Geometry: final body of the model. Coordinates: model frame, mm. A direction names the side the tool comes from. Coordinates: 2 decimals unless noted, no trailing zeros. Write each loop counter-clockwise with the first axis right and the second up, starting at its lowest first coordinate (ties: lowest second). Pieces come first, ordered by that corner, then holes. Notation, with made-up numbers: (27.25, 78.25) - (62.25, 78.25) arc R13 cw to (62.25, 85.25) - close; hole circle Ø3 at (-15.75, 18). An arc over 180 degrees is marked (long way). Put each result on its own line as item: value.
```python
from build123d import *

# Parameters (mm, degrees)
ESQUISSE5_W         = 84
ESQUISSE5_H         = 56
BOSS_EXTRU_6_DEPTH  = 1.6
ESQUISSE6_W         = 77
ESQUISSE6_H         = 54
BOSS_EXTRU_8_DEPTH  = 3.5
ESQUISSE8_W         = 4
ESQUISSE8_H         = 6
BOSS_EXTRU_10_DEPTH = 1.5
ESQUISSE7_W         = 4
ESQUISSE7_H         = 6
BOSS_EXTRU_11_DEPTH = 1.5
ESQUISSE11_W        = 4
ESQUISSE11_H        = 6
BOSS_EXTRU_12_DEPTH = 1.5


with BuildPart() as part:
    # Esquisse5 → Boss.-Extru.6 (new body)
    with BuildSketch(Plane.XY):
        with Locations((42, 28)):
            Rectangle(ESQUISSE5_W, ESQUISSE5_H)
    extrude(amount=BOSS_EXTRU_6_DEPTH)

    # Esquisse6 → Boss.-Extru.8 (add)
    with BuildSketch(Plane(origin=(0, 0, 0), x_dir=(-1, 0, 0), z_dir=(0, 0, -1))):
        with Locations((-39.5, 28)):
            Rectangle(ESQUISSE6_W, ESQUISSE6_H)
    extrude(amount=BOSS_EXTRU_8_DEPTH)

    # Esquisse8 → Boss.-Extru.10 (add)
    with BuildSketch(Plane(origin=(0, 0, 0), x_dir=(-1, 0, 0), z_dir=(0, 0, -1))):
        with Locations((-81, 26)):
            Rectangle(ESQUISSE8_W, ESQUISSE8_H)
    extrude(amount=BOSS_EXTRU_10_DEPTH)

    # Esquisse7 → Boss.-Extru.11 (add)
    with BuildSketch(Plane(origin=(0, 0, 0), x_dir=(-1, 0, 0), z_dir=(0, 0, -1))):
        with Locations((-81, 39)):
            Rectangle(ESQUISSE7_W, ESQUISSE7_H)
    extrude(amount=BOSS_EXTRU_11_DEPTH)

    # Esquisse11 → Boss.-Extru.12 (add)
    with BuildSketch(Plane(origin=(0, 0, 0), x_dir=(-1, 0, 0), z_dir=(0, 0, -1))):
        with Locations((-81, 13)):
            Rectangle(ESQUISSE11_W, ESQUISSE11_H)
    extrude(amount=BOSS_EXTRU_12_DEPTH)


solid = part.part
```
1. Section query D-D (y = 14). Return loops of the section in (x, z).
Answer below:
outline: (0, 0) - (1, 0) - (1, -3.5) - (78, -3.5) - (78, 0) - (79, 0) - (79, -1.5) - (83, -1.5) - (83, 0) - (84, 0) - (84, 1.6) - (0, 1.6) - close
2. Section query A-A (y = 51.5). Return loops of the section in (x, z).
Answer below:
outline: (0, 0) - (1, 0) - (1, -3.5) - (78, -3.5) - (78, 0) - (84, 0) - (84, 1.6) - (0, 1.6) - close
3. Mould query, pull axis X, two halves, no side actions, for faces 4 (the flat face through (1, 28, -2)), 5 (the flat face through (78, 28, -2)), 6 (the flat face through (41, 28, 1.6)). Classes: +X half, -X half, draft (parallel to the pull), parting line (faces both ways), or undercut.
Answer below:
face 4: -X half
face 5: undercut
face 6: draft
4. Section query B-B (x = 51.5). Return loops of the section in (y, z), then the cut area to 3 significant figures.
Answer below:
outline: (0, 0) - (1, 0) - (1, -3.5) - (55, -3.5) - (55, 0) - (56, 0) - (56, 1.6) - (0, 1.6) - close
area: 279 mm²
5. Set-up query: faces 1 (the flat face through (40, 1, -2)), 2 (the flat face through (40, 55, -2)), 3 (the flat face through (81, 39, -1.5)). Return all of +Z, -Z, +X, -X, +Y, -Y with unobstructed straight access to the full face (end or side cutting, diameter ignored); none if empty.
Answer below:
face 1: -Z, +X, -X, -Y
face 2: -Z, +X, -X, +Y
face 3: -Z, +X, +Y, -Y
6. Section query C-C (z = -2.45). Return loops of the section in (x, y), then the cut area to 3 significant figures.
Answer below:
outline: (1, 1) - (78, 1) - (78, 55) - (1, 55) - close
area: 4,160 mm²
7. Ray query, probe 1 along X at (y, z) = (39.5, -0.6); probe 2 along Y at (x, z) = (63, -0.5); probe 3 along X at (y, z) = (35, -1). Return the intervals inside material, ascending. Write a range as from..to.
Answer below:
probe 1: x = 1..78, 79..83
probe 2: y = 1..55
probe 3: x = 1..78
8. Pin query (flat end, axial travel): pin 1 Ø1 at (x, z) = (45, -2) entering from -Y; pin 2 Ø1 at (y, z) = (19.5, -2) entering from +X; pin 3 Ø4.5 at (x, y) = (80.5, 26) entering from -Z. Return the tip coordinate at first contact, or that it passes through.
Answer below:
pin 1: stops at y = 1
pin 2: stops at x = 78
pin 3: stops at z = -1.5
